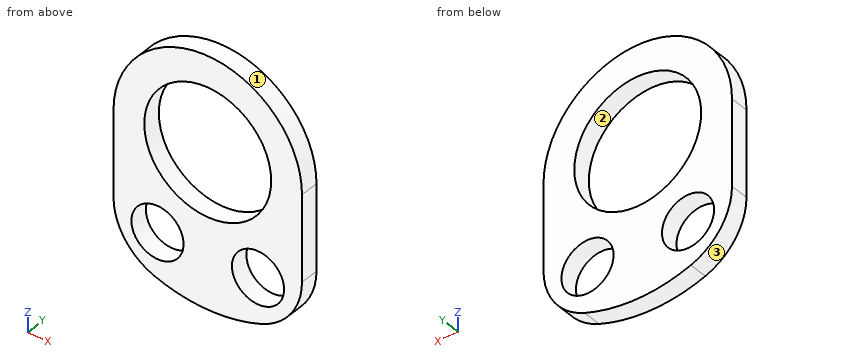
Autodesk Inventor part; units mm, degrees
ref_plane "YZ Plane" through (0, 0, 0) normal (1, 0, 0) x (0, 1, 0)
ref_plane "XZ Plane" through (0, 0, 0) normal (0, 1, 0) x (-1, 0, 0)
ref_plane "XY Plane" through (0, 0, 0) normal (0, 0, 1) x (1, 0, 0)
sketch "Sketch1" plane through (0, 0, 0) normal (0, 1, 0) x (-1, 0, 0)
  circle A0 centre (0, 0) radius 10.1
  circle A1 centre (8, -16) radius 4.15
  circle A2 centre (-8, -16) radius 4.15
  circle A3 centre (0, 0) radius 24.4957
  line L0 (15, 0) -> (15, -19.3659)
  line L1 (-15, 0) -> (-15, -19.3659)
  arc A4 (15, 0) -> (-15, 0) centre (0, 0) ccw
  arc A5 (-9.0276, -11.9792) -> (-4.1668, -14.4096) centre (0, 0) ccw
  dimension "d0" = 20.2
  dimension "d1" = 8.3
  dimension "d2" = 8.3
  dimension "d3" = 16
  dimension "d4" = 16
  dimension "d5" = 16
  dimension "d6" = 8
extrude "Extrusion1" add sketch "Sketch1" along normal blind 3 contours L1 A4 L0 A3 picked at (13.8916, -11.1458)
fillet "Fillet1" radius 10 2 edges at (15, 1.5, -19.3659) (-15, 1.5, -19.3659)
equation "\"d2\" = d1"
properties part number "Sujeción mangueras_3DPrint"
Could you check a few things on this model? Use its own coordinates, in mm. Face numbers are marked on the shaded views. Coordinates: 2 decimals unless noted, no trailing zeros. Loops run counter-clockwise (first coordinate to the right, second up) from the corner with the lowest first, then second, coordinate; pieces in that order, holes last.
1. Imagine slicing it at D-D (z = -16). Please give me the cut outline in (x, y), and give its area (3 significant figures).
2. Imagine slicing it at C-C (y = 1.5). Please give me the cut outline in (x, z), and give its area (3 significant figures).
3. Imagine slicing it at A-A (z = -2). Please give me the cut outline in (x, y), and give its area (3 significant figures).
4. I need wall thicknesses on L1, parallel to Z at x = -8, y = 2.05; L2, parallel to Z at x = -7.25, y = 1.65; L3, parallel to Z at x = 0, y = 1.8. Which ranges of each line are inside material? Lowest first, please.
5. We'd pull the mould along X, two halves only. Please class the marked faces 1, 2 and 3: released by +X, released by -X, zero draft, split by the parting line, or undercut.
6. Imagine slicing it at B-B (x = 0). Please give me the cut outline in (y, z), and give its area (3 significant figures).
Computed values:
1. outline: (-14.71, 0) - (-12.15, 0) - (-12.15, 3) - (-14.71, 3) - close; (-3.85, 0) - (3.85, 0) - (3.85, 3) - (-3.85, 3) - close; (12.15, 0) - (14.71, 0) - (14.71, 3) - (12.15, 3) - close
1. area: 38.5 mm2
2. outline: (-15, -13.61) arc R10 ccw to (-8.45, -22.99) arc R24.5 ccw to (8.45, -22.99) arc R10 ccw to (15, -13.61) - (15, 0) arc R15 ccw to (-15, 0) - close; hole circle Ø8.3 at (-8, -16); hole circle Ø20.2 at (0, 0); hole circle Ø8.3 at (8, -16)
2. area: 598 mm2
3. outline: (-15, 0) - (-9.9, 0) - (-9.9, 3) - (-15, 3) - close; (9.9, 0) - (15, 0) - (15, 3) - (9.9, 3) - close
3. area: 30.6 mm2
4. L1: z = -23.15 to -20.15, -11.85 to -6.17, 6.17 to 12.69
4. L2: z = -23.4 to -20.08, -11.92 to -7.03, 7.03 to 13.13
4. L3: z = -24.5 to -10.1, 10.1 to 15
5. face 1: split by the parting line
5. face 2: undercut
5. face 3: released by -X
6. outline: (0, -24.5) - (3, -24.5) - (3, -10.1) - (0, -10.1) - close; (0, 10.1) - (3, 10.1) - (3, 15) - (0, 15) - close
6. area: 57.9 mm2
